Verification items for the finished model (mm, model axes). Face numbers are marked on the shaded views. A direction names the side the tool comes from. Give positions to 0.01 mm unless a question says otherwise; leave off trailing zeros. Order: outer loops, then holes, each group sorted by start corner. A loop starts at its lowest first (then second) coordinate and runs counter-clockwise, first axis right, second up.
(1) Sectioned sample at B-B on x = 0. Record the cut outline in (y, z), plus the area to 3 significant figures.
(2) Gauge pin test, flat ends, axial feed: pin 1 (3 mm diameter, centred on y = 15.5, z = -5.5, fed in from +X); pin 2 (3 mm diameter, centred on x = 9.5, z = -6.5, fed in from -Y); pin 3 (1 mm diameter, centred on x = -3.5, y = 4.5, fed in from +Z). Record the tip position at first contact, or that the pin passes through.
(3) Scan lines: L1, parallel to Y at x = 3.5, z = -7; L2, parallel to Y at x = -4.5, z = -4.75; L3, parallel to X at y = 17.75, z = -11. Record each from-to range of solid material in increasing order.
(4) Sectioned sample at A-A on z = 0. Record the cut outline in (x, y), plus the area to 3 significant figures.
(5) Sectioned sample at C-C on y = 9.5. Record the cut outline in (x, z).
(6) Access from +Z, -Z, +X, -X, +Y, -Y to the whole of each face (thin tool, end or side, straight path). Record for the marked faces 3 and 4.
(7) Mould release check, pull along X, two halves, no side actions. Record for the marked faces 1 and 2: pulls with the +X half, pulls with the -X half, needs draft (parallel to the pull), parting line crosses it, or undercut.
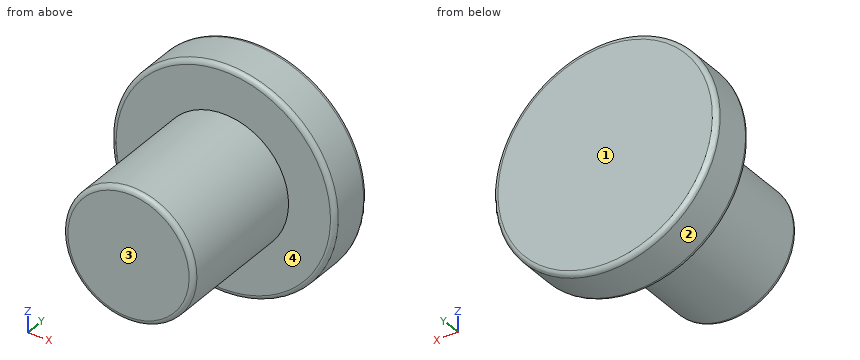
```python
from build123d import *

# Parameters (mm, degrees)
FILETE1_R = 0.5


with BuildPart() as part:
    # Esboço1 → Revolução1 (revolve)
    with BuildSketch(Plane.XY, mode=Mode.PRIVATE) as revolu_o1_sk:
        Polygon((0, 0), (0, 20), (12, 20), (12, 15), (7, 15), (7, 0), align=None)
    revolve(revolu_o1_sk.sketch.rotate(Axis((0, 0, 0), (0, 1, 0)), 90), axis=Axis((0, 0, 0), (0, 1, 0)))  # turned: the seam where the file's is

    # Filete1
    filete1_edges = [part.edges().sort_by_distance(p)[0] for p in [
        (0, 0, 7),
        (0, 15, 12),
        (0, 20, 12),
    ]]
    fillet(filete1_edges, radius=FILETE1_R)


solid = part.part
```
Ans:
1. outline: (0, -6.5) arc R0.5 ccw to (0.5, -7) - (15, -7) - (15, -11.5) arc R0.5 ccw to (15.5, -12) - (19.5, -12) arc R0.5 ccw to (20, -11.5) - (20, 11.5) arc R0.5 ccw to (19.5, 12) - (15.5, 12) arc R0.5 ccw to (15, 11.5) - (15, 7) - (0.5, 7) arc R0.5 ccw to (0, 6.5) - close
1. area: 330 mm2
2. pin 1: stops at x = 11.31
2. pin 2: stops at y = 15
2. pin 3: stops at z = 6.32
3. L1: y = 15 to 20
3. L2: y = 0 to 20
3. L3: x = -4.8 to 4.8
4. outline: (-12, 15.5) arc R0.5 ccw to (-11.5, 15) - (-7, 15) - (-7, 0.5) arc R0.5 ccw to (-6.5, 0) - (6.5, 0) arc R0.5 ccw to (7, 0.5) - (7, 15) - (11.5, 15) arc R0.5 ccw to (12, 15.5) - (12, 19.5) arc R0.5 ccw to (11.5, 20) - (-11.5, 20) arc R0.5 ccw to (-12, 19.5) - close
4. area: 330 mm2
5. outline: circle Ø14 at (0, 0)
6. face 3: +Z, -Z, +X, -X, -Y
6. face 4: -Y
7. face 1: needs draft
7. face 2: parting line crosses it
